The figure shows three views and two pictorial views of one solid part (mm, origin at its lowest corner). Answer the questions. A direction names the side the tool comes from. Coordinates: 2 decimals unless noted, no trailing zeros. Order: outer loops, then holes, each group sorted by start corner. A loop starts at its lowest first (then second) coordinate and runs counter-clockwise, first axis right, second up. Notation, with made-up numbers: (72, 65) - (77, 65) arc R17 ccw to (77, 93) - close; hole circle Ø4 at (62, 51). An arc over 180 degrees is marked (long way). Use one line per item in the form item = value. Start each with the question number.
Item 1: Each of these flat-tipped pins is pushed along its axis until it touches: pin 1 Ø4 at (y, z) = (3, 8) entering from +X (1 decimal); pin 2 Ø12 at (x, z) = (62, 14.5) entering from +Y; pin 3 Ø3 at (x, y) = (16.5, 5.5) entering from -Z. Where does it stop, or does it pass through?
Item 2: Section D-D, the plane x = 59 is taken. Write down the section's boundary in (y, z), and give its area (3 significant figures).
Item 3: Consider line 1 along X through (y, z) = (2, 19.5); line 2 along Z through (x, y) = (8.5, 6) (1 decimal); line 3 along Y through (x, z) = (62.5, 47.5). Determine where each line is inside the solid, lowest interval first. Write a range as [from, to].
Item 4: Section C-C, the plane z = 35 is taken. Write down the section's boundary in (x, y), and give its area (3 significant figures).
Item 5: Section B-B, the plane y = 2.5 is taken. Write down the section's boundary in (x, z).
Item 6: A tool of negligible diameter and unlimited length cuts with its end or side. For the marked faces 1 and 2, from which of +Z, -Z, +X, -X, +Y, -Y can it reach the whole face along a straight path? Write none if from no direction.
Item 7: Section A-A, the plane z = 19.5 is taken. Write down the section's boundary in (x, y) (1 decimal), and give its area (3 significant figures).
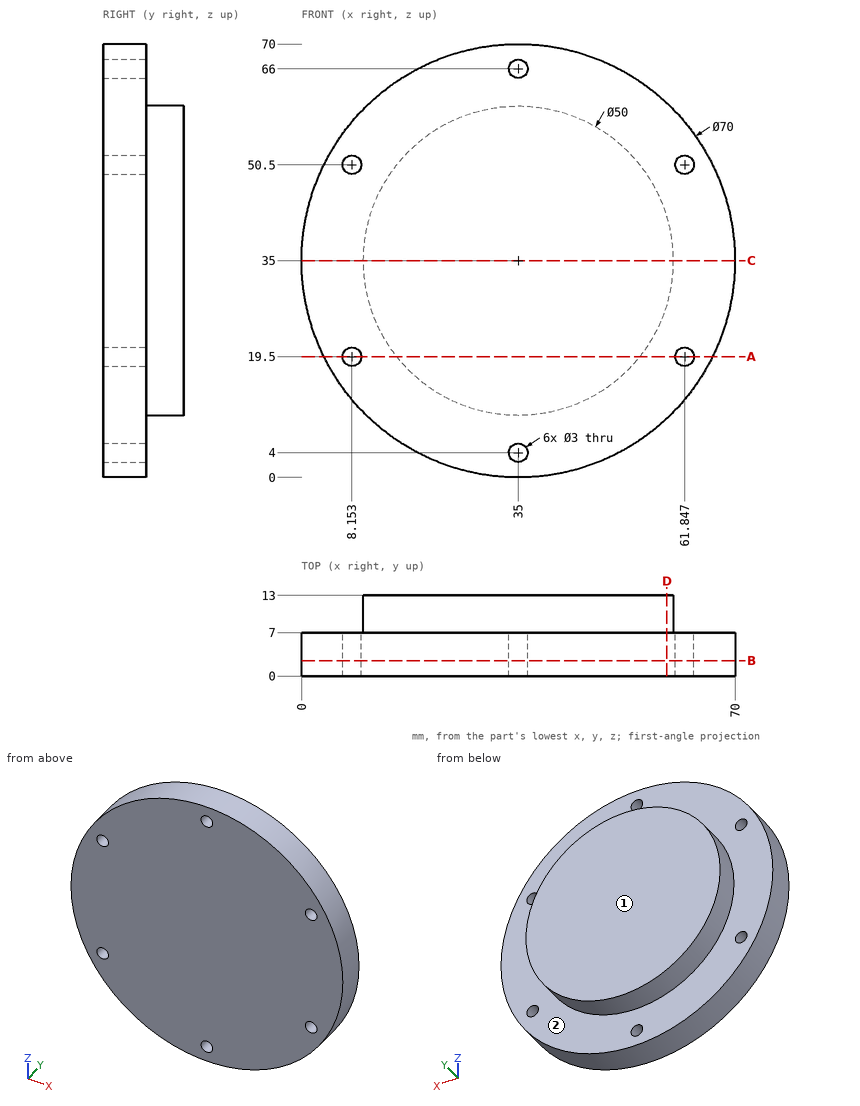
Response:
q1.pin_1 = 59.5
q1.pin_2 = 7
q1.pin_3 = 4.41
q2.outline = (0, 9.52) - (7, 9.52) - (7, 28) - (13, 28) - (13, 42) - (7, 42) - (7, 60.48) - (0, 60.48) - close
q2.area = 441 mm2
q3.line_1 = [3.62, 6.65], [9.65, 60.35], [63.35, 66.38]
q3.line_2 = [12.1, 18], [21, 49], [52, 57.9]
q3.line_3 = [0, 7]
q4.outline = (0, 0) - (70, 0) - (70, 7) - (60, 7) - (60, 13) - (10, 13) - (10, 7) - (0, 7) - close
q4.area = 790 mm2
q5.outline = circle Ø70 at (35, 35); hole circle Ø3 at (8.15, 19.5); hole circle Ø3 at (8.15, 50.5); hole circle Ø3 at (35, 4); hole circle Ø3 at (35, 66); hole circle Ø3 at (61.85, 19.5); hole circle Ø3 at (61.85, 50.5)
q6.face_1 = +Z, -Z, +X, -X, +Y
q6.face_2 = +Y
q7.outline = (3.6, 0) - (6.7, 0) - (6.7, 7) - (3.6, 7) - close; (9.7, 0) - (60.3, 0) - (60.3, 7) - (54.6, 7) - (54.6, 13) - (15.4, 13) - (15.4, 7) - (9.7, 7) - close; (63.3, 0) - (66.4, 0) - (66.4, 7) - (63.3, 7) - close
q7.area = 633 mm2
